Model file for the job. Use its own axes, mm. A direction names the side the tool comes from. Coordinates: 2 decimals unless noted, no trailing zeros. Order: outer loops, then holes, each group sorted by start corner. A loop starts at its lowest first (then second) coordinate and runs counter-clockwise, first axis right, second up. Notation, with made-up numbers: (18.25, -11.5) -> (53.25, -11.5) arc R7 ccw to (53.25, 0.5) -> close; hole circle Ø9 at (-12.5, -33.5). An arc over 180 degrees is marked (long way). Return JSON: item names as keys, results as strings. Group by question number.
1) Pull direction X, two halves, no side cores. Call faces 6 (the flat face through (4, 0, -10)), 7 (the cylindrical face through (-47.34, 9.13, -5.74)), 8 (the flat face through (-114.3, 8.9, 1.6)): +X half, -X half, draft (parallel to the pull), parting line (faces both ways), or undercut.
2) Cut at C-C (z = -19.25). Write the cut outline in (x, y).
3) Cut at B-B (z = -5.2). Write the cut outline in (x, y), and give its area (3 significant figures).
4) Cut at A-A (x = 4.7). Write the cut outline in (y, z).
5) Flat gauge pins, fed straight in: pin 1 (5 mm diameter, centred on x = -47.5, z = -3.5, fed in from -Y); pin 2 (3 mm diameter, centred on x = 4.7, z = -15.2, fed in from +Y); pin 3 (3 mm diameter, centred on x = 4.5, y = 10, fed in from +Z). Where does each tip first touch, or does it go through?
6) Which spindle directions (+Z, -Z, +X, -X, +Y, -Y) get a long thin tool onto all of the face, cutting with end or side? Do faces 1 (the cylindrical face through (3.74, 9.13, -2.89)), 2 (the flat face through (0, 9, -10)), 3 (the flat face through (-104.9, 8.9, -13)), 4 (the flat face through (-91, 9, 3)), 5 (the flat face through (3, 9, 0)). Say none if no direction does.
7) Cut at D-D (x = -10.1). Write the cut outline in (y, z).
8) Probe line 1 (X direction, y = 4.25, z = -5.2); line 2 (X direction, y = 13.5, z = -17); line 3 (Z direction, x = 2.5, y = -7.5). List the from-to ranges inside material, lowest first.
from build123d import *

# Parameters (mm, degrees)
BOSS_EXTRUDE1_DEPTH = 18
SKETCH2_W           = 52
SKETCH2_H           = 29
BOSS_EXTRUDE2_DEPTH = 4
SKETCH3_W           = 52
SKETCH3_H           = 24.4
BOSS_EXTRUDE3_DEPTH = 4
SKETCH4_R           = 2.5
BOSS_EXTRUDE4_DEPTH = 5
SKETCH5_R           = 2.5
CUT_EXTRUDE1_DEPTH  = 18
FILLET2_R           = 6
FILLET4_R           = 2
FILLET5_R           = 100


with BuildPart() as part:
    # Sketch1 → Boss-Extrude1 (new body)
    with BuildSketch(Plane(origin=(0, 0, 0), x_dir=(1, 0, 0), z_dir=(0, 1, 0))):
        with BuildLine():
            Line((-40.2, 0), (-40.2, 20.4))
            Line((-40.2, 20.4), (0, 20.4))
            Line((0, 20.4), (0, 0))
            Line((0, 0), (8, 0))
            Line((8, 0), (8, 24.4))
            Line((8, 24.4), (-44, 24.4))
            Line((-44, 24.4), (-54, 14.4))
            Line((-54, 14.4), (-104, 14.4))
            Line((-104, 14.4), (-105.811278075, 11.586050134))
            ThreePointArc((-105.811278075, 11.586050134), (-115.486050134, 9.488721925), (-113.388721925, -0.186050134))
            Line((-113.388721925, -0.186050134), (-115.2, -3))
            Line((-115.2, -3), (-55.2, -3))
            Line((-55.2, -3), (-40.2, 0))
        make_face()
    extrude(amount=BOSS_EXTRUDE1_DEPTH)

    # Sketch2 → Boss-Extrude2 (add)
    with BuildSketch(Plane(origin=(0, 0, -24.4), x_dir=(-1, 0, 0), z_dir=(0, 0, -1))):
        with Locations((18, 3.5)):
            Rectangle(SKETCH2_W, SKETCH2_H)
    extrude(amount=-BOSS_EXTRUDE2_DEPTH)

    # Sketch3 → Boss-Extrude3 (add)
    with BuildSketch(Plane.XZ.offset(11)):
        with Locations((-18, -12.2)):
            Rectangle(SKETCH3_W, SKETCH3_H)
    extrude(amount=BOSS_EXTRUDE3_DEPTH)

    # Sketch4 → Boss-Extrude4 (add)
    with BuildSketch(Plane.XZ.offset(15)):
        with Locations(Location((-10.1, -10.2, 0), (0, 0, 270))):
            Circle(SKETCH4_R)
    extrude(amount=BOSS_EXTRUDE4_DEPTH)

    # Sketch5 → Cut-Extrude1 (cut)
    with BuildSketch(Plane(origin=(0, 18, 0), x_dir=(1, 0, 0), z_dir=(0, 1, 0))):
        with Locations(Location((4.7, 15.2, 0), (0, 0, 270))):
            Circle(SKETCH5_R)
        with Locations(Location((4.7, 5.2, 0), (0, 0, 270))):
            Circle(SKETCH5_R)
        with Locations(Location((-44.9, 5.2, 0), (0, 0, 270))):
            Circle(SKETCH5_R)
        with Locations(Location((-44.9, 15.2, 0), (0, 0, 270))):
            Circle(SKETCH5_R)
    extrude(amount=-CUT_EXTRUDE1_DEPTH, mode=Mode.SUBTRACT)

    # Fillet2
    fillet2_edges = [part.edges().sort_by_distance(p)[0] for p in [
        (-54, 9, -14.4),
    ]]
    fillet(fillet2_edges, radius=FILLET2_R)

    # Fillet4
    fillet4_edges = [part.edges().sort_by_distance(p)[0] for p in [
        (8, 1.5, -24.4),
        (8, 9, 0),
        (8, -13, 0),
    ]]
    fillet(fillet4_edges, radius=FILLET4_R)

    # Fillet5
    fillet5_edges = [part.edges().sort_by_distance(p)[0] for p in [
        (-55.2, 9, 3),
    ]]
    fillet(fillet5_edges, radius=FILLET5_R)


solid = part.part
Answers below:
{
 "1": {"face 6": "draft", "face 7": "undercut", "face 8": "-X half"},
 "2": {"outline": "(-49.15, 0) -> (-40.2, 0) -> (-40.2, 18) -> (-49.15, 18) -> close; (-44, -15) -> (8, -15) -> (8, -11) -> (-44, -11) -> close; (0, 0) -> (8, 0) -> (8, 18) -> (0, 18) -> close"},
 "3": {"outline": "(-116.58, 0) -> (-47.4, 0) -> (-47.4, 18) -> (-116.58, 18) -> close; (-44, -15) -> (8, -15) -> (8, -11) -> (-44, -11) -> close; (-42.4, 0) -> (-40.2, 0) -> (-40.2, 18) -> (-42.4, 18) -> close; (0, 0) -> (2.2, 0) -> (2.2, 18) -> (0, 18) -> close; (7.2, 0) -> (8, 0) -> (8, 18) -> (7.2, 18) -> close", "area": "1,550 mm^2"},
 "4": {"outline": "(-15, -24.4) -> (18, -24.4) -> (18, -17.7) -> (0, -17.7) -> (0, -20.4) -> (-11, -20.4) -> (-11, 0) -> (-15, 0) -> close; (0, -12.7) -> (18, -12.7) -> (18, -7.7) -> (0, -7.7) -> close; (0, -2.7) -> (18, -2.7) -> (18, 0) -> (0, 0) -> close"},
 "5": {"pin 1": "stops at y = 0", "pin 2": "stops at y = -11", "pin 3": "stops at z = 0"},
 "6": {"face 1": "+Y", "face 2": "+Z, +Y", "face 3": "-Z, +Y, -Y", "face 4": "+Z, +X, -X, +Y, -Y", "face 5": "+Z, +X, +Y, -Y"},
 "7": {"outline": "(-20, -12.7) -> (-15, -12.7) -> (-15, -24.4) -> (18, -24.4) -> (18, -20.4) -> (-11, -20.4) -> (-11, 0) -> (-15, 0) -> (-15, -7.7) -> (-20, -7.7) -> close"},
 "8": {"line 1": "x = -116.58 to -47.4, -42.4 to -40.2, 0 to 2.2, 7.2 to 8", "line 2": "x = -51.4 to -46.63, -43.17 to -40.2, 0 to 2.97, 6.43 to 8", "line 3": "z = -24.4 to -20.4"}
}
